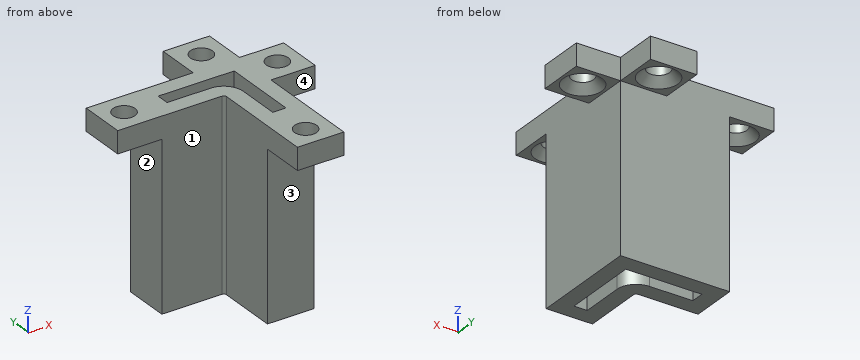
```python
from build123d import *

# Parameters (mm, degrees)
BOSS_EXTRUDE1_DEPTH = 30
BOSS_EXTRUDE2_DEPTH = 4
SKETCH4_R           = 2
CUT_EXTRUDE1_DEPTH  = 4
CHAMFER1_SIZE       = 1.5


with BuildPart() as part:
    # Sketch2 → Boss-Extrude1 (new body)
    with BuildSketch(Plane.XY.offset(10)):
        with BuildLine():
            Line((-14.944066591, 82.328103542), (-14.944066591, 62.528103542))
            Line((-14.944066591, 62.528103542), (-23.344066591, 62.528103542))
            Line((-23.344066591, 62.528103542), (-23.344066591, 73.428103542))
            ThreePointArc((-23.344066591, 73.428103542), (-23.490513201, 73.781656932), (-23.844066591, 73.928103542))
            Line((-23.844066591, 73.928103542), (-34.744066591, 73.928103542))
            Line((-34.744066591, 73.928103542), (-34.744066591, 82.328103542))
            Line((-34.744066591, 82.328103542), (-14.944066591, 82.328103542))
        make_face()
        with BuildLine():
            Line((-17.944066591, 79.328103542), (-17.944066591, 65.528103542))
            Line((-17.944066591, 65.528103542), (-20.344066591, 65.528103542))
            Line((-20.344066591, 65.528103542), (-20.344066591, 73.428103542))
            ThreePointArc((-20.344066591, 73.428103542), (-21.369192857, 75.902977276), (-23.844066591, 76.928103542))
            Line((-23.844066591, 76.928103542), (-31.744066591, 76.928103542))
            Line((-31.744066591, 76.928103542), (-31.744066591, 79.328103542))
            Line((-31.744066591, 79.328103542), (-17.944066591, 79.328103542))
        make_face(mode=Mode.SUBTRACT)
    extrude(amount=BOSS_EXTRUDE1_DEPTH)

    # Sketch3 → Boss-Extrude2 (add)
    with BuildSketch(Plane.XY.offset(40)):
        with BuildLine():
            Line((-34.744066591, 82.328103542), (-42.744066591, 82.328103542))
            Line((-42.744066591, 82.328103542), (-42.744066591, 73.928103542))
            Line((-42.744066591, 73.928103542), (-34.744066591, 73.928103542))
            Line((-34.744066591, 73.928103542), (-23.844066591, 73.928103542))
            ThreePointArc((-23.844066591, 73.928103542), (-23.490513201, 73.781656932), (-23.344066591, 73.428103542))
            Line((-23.344066591, 73.428103542), (-23.344066591, 62.528103542))
            Line((-23.344066591, 62.528103542), (-23.344066591, 54.528103542))
            Line((-23.344066591, 54.528103542), (-14.944066591, 54.528103542))
            Line((-14.944066591, 54.528103542), (-14.944066591, 62.528103542))
            Line((-14.944066591, 62.528103542), (-14.944066591, 73.928103542))
            Line((-14.944066591, 73.928103542), (-6.944066591, 73.928103542))
            Line((-6.944066591, 73.928103542), (-6.944066591, 82.328103542))
            Line((-6.944066591, 82.328103542), (-14.944066591, 82.328103542))
            Line((-14.944066591, 82.328103542), (-14.944066591, 90.328103542))
            Line((-14.944066591, 90.328103542), (-23.344066591, 90.328103542))
            Line((-23.344066591, 90.328103542), (-23.344066591, 82.328103542))
            Line((-23.344066591, 82.328103542), (-34.744066591, 82.328103542))
        make_face()
        with BuildLine():
            Line((-31.744066591, 76.928103542), (-23.844066591, 76.928103542))
            ThreePointArc((-23.844066591, 76.928103542), (-21.369192857, 75.902977276), (-20.344066591, 73.428103542))
            Line((-20.344066591, 73.428103542), (-20.344066591, 65.528103542))
            Line((-20.344066591, 65.528103542), (-17.944066591, 65.528103542))
            Line((-17.944066591, 65.528103542), (-17.944066591, 79.328103542))
            Line((-17.944066591, 79.328103542), (-31.744066591, 79.328103542))
            Line((-31.744066591, 79.328103542), (-31.744066591, 76.928103542))
        make_face(mode=Mode.SUBTRACT)
    extrude(amount=BOSS_EXTRUDE2_DEPTH)

    # Sketch4 → Cut-Extrude1 (cut)
    with BuildSketch(Plane(origin=(0, 0, 40), x_dir=(-1, 0, 0), z_dir=(0, 0, -1))):
        with Locations((19.144066591, 86.328103542)):
            Circle(SKETCH4_R)
        with Locations((10.944066591, 78.128103542)):
            Circle(SKETCH4_R)
        with Locations((38.744066591, 78.128103542)):
            Circle(SKETCH4_R)
        with Locations((19.144066591, 58.528103542)):
            Circle(SKETCH4_R)
    extrude(amount=-CUT_EXTRUDE1_DEPTH, mode=Mode.SUBTRACT)

    # Chamfer1
    chamfer1_edges = [part.edges().sort_by_distance(p)[0] for p in [
        (-17.144066591, 86.328103542, 40),
        (-8.944066591, 78.128103542, 40),
        (-36.744066591, 78.128103542, 40),
        (-17.144066591, 58.528103542, 40),
    ]]
    chamfer(chamfer1_edges, length=CHAMFER1_SIZE)


solid = part.part
```
Read the model definition and answer for the solid it produces. Units are mm, in the model's axes. Face numbers are marked on the shaded views. A direction names the side the tool comes from. Coordinates: 2 decimals unless noted, no trailing zeros. Loops run counter-clockwise (first coordinate to the right, second up) from the corner with the lowest first, then second, coordinate; pieces in that order, holes last. Notation, with made-up numbers: (80.25, 44.25) - (125.25, 44.25) arc R23 ccw to (125.25, 70.25) - close; hole circle Ø2 at (17.25, 5.25). An arc over 180 degrees is marked (long way). Answer in a Markdown table with one row per item.
1. Find section B-B, the plane z = 23. Write down the section's boundary in (x, y).
Conclusion:
| item | result |
|---|---|
| outline | (-34.74, 73.93) - (-23.84, 73.93) arc R0.5 cw to (-23.34, 73.43) - (-23.34, 62.53) - (-14.94, 62.53) - (-14.94, 82.33) - (-34.74, 82.33) - close; hole (-31.74, 76.93) - (-23.84, 76.93) arc R3.5 cw to (-20.34, 73.43) - (-20.34, 65.53) - (-17.94, 65.53) - (-17.94, 79.33) - (-31.74, 79.33) - close |
2. Find section D-D, the plane y = 64.5. Write down the section's boundary in (x, z).
Conclusion:
| item | result |
|---|---|
| outline | (-23.34, 10) - (-14.94, 10) - (-14.94, 44) - (-23.34, 44) - close |
3. Find section C-C, the plane z = 40.5. Write down the section's boundary in (x, y).
Conclusion:
| item | result |
|---|---|
| outline | (-42.74, 73.93) - (-23.84, 73.93) arc R0.5 cw to (-23.34, 73.43) - (-23.34, 54.53) - (-14.94, 54.53) - (-14.94, 73.93) - (-6.94, 73.93) - (-6.94, 82.33) - (-14.94, 82.33) - (-14.94, 90.33) - (-23.34, 90.33) - (-23.34, 82.33) - (-42.74, 82.33) - close; hole circle Ø6 at (-38.74, 78.13); hole (-31.74, 76.93) - (-23.84, 76.93) arc R3.5 cw to (-20.34, 73.43) - (-20.34, 65.53) - (-17.94, 65.53) - (-17.94, 79.33) - (-31.74, 79.33) - close; hole circle Ø6 at (-19.14, 58.53); hole circle Ø6 at (-19.14, 86.33); hole circle Ø6 at (-10.94, 78.13) |
4. Straight lines are drawn through the part: line 1 (X direction, y = 77.5, z = 35.5); line 2 (X direction, y = 69.5, z = 29); line 3 (Y direction, x = -18, z = 25.5). For each, find the intervals that lie inside material, in ascending order.
Conclusion:
| item | result |
|---|---|
| line 1 | x = -34.74 to -31.74, -17.94 to -14.94 |
| line 2 | x = -23.34 to -20.34, -17.94 to -14.94 |
| line 3 | y = 62.53 to 65.53, 79.33 to 82.33 |
5. Find section A-A, the plane y = 72. Write down the section's boundary in (x, z), then the cut area to 3 significant figures.
Conclusion:
| item | result |
|---|---|
| outline | (-23.34, 10) - (-20.34, 10) - (-20.34, 44) - (-23.34, 44) - close; (-17.94, 10) - (-14.94, 10) - (-14.94, 44) - (-17.94, 44) - close |
| area | 204 mm² |
6. Which of the six approach directions +Z, -Z, +X, -X, +Y, -Y give full straight-line access (tool end or side, diameter ignored) to the marked faces 1, 2, 3 and 4?
Conclusion:
| item | result |
|---|---|
| face 1 | +Z, -Z, -X, -Y |
| face 2 | -Z, -X, +Y, -Y |
| face 3 | -Z, +X, -X, -Y |
| face 4 | +Z, -Z, +X, -Y |
7. Given pin 1 (5 mm diameter, centred on x = -10.94, y = 78.13, fed in from -Z); pin 2 (3 mm diameter, centred on y = 86, z = 42.5, fed in from +X); pin 3 (1.5 mm diameter, centred on x = -26.5, z = 36, fed in from +Y), each flat-ended and moving along its own axis, determine where each tip first touches the part or whether it passes through.
Conclusion:
| item | result |
|---|---|
| pin 1 | stops at z = 41 |
| pin 2 | stops at x = -14.94 |
| pin 3 | stops at y = 82.33 |
